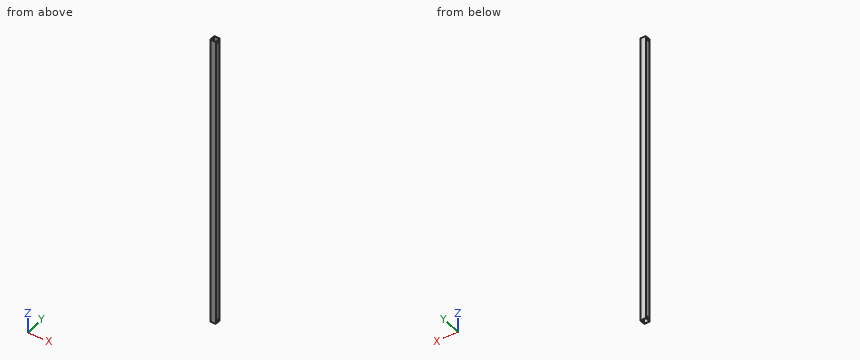
Autodesk Inventor part; units mm, degrees
ref_plane "YZ Plane" through (0, 0, 0) normal (1, 0, 0) x (0, 1, 0)
ref_plane "XZ Plane" through (0, 0, 0) normal (0, 1, 0) x (-1, 0, 0)
ref_plane "XY Plane" through (0, 0, 0) normal (0, 0, 1) x (1, 0, 0)
sketch "Sketch1" plane through (0, 0, 0) normal (0, 0, 1) x (1, 0, 0)
  line L0 (-12.7, 12.7) -> (12.7, 12.7)
  line L1 (12.7, 12.7) -> (12.7, -12.7)
  line L2 (12.7, -12.7) -> (-12.7, -12.7)
  line L3 (-12.7, -12.7) -> (-12.7, 12.7)
  line L4 (-17.78, 0) -> (17.78, 0)
  line L5 (0, 17.78) -> (0, -17.78)
  line L6 (11.43, 11.43) -> (-11.43, 11.43)
  line L7 (-11.43, 11.43) -> (-11.43, -11.43)
  line L8 (-11.43, -11.43) -> (11.43, -11.43)
  line L9 (11.43, -11.43) -> (11.43, 11.43)
  point P0 (0, 0)
  dimension "d0" = 25.4
  dimension "d1" = 1.27
extrude "Extrusion1" add sketch "Sketch1" along normal mid plane 1384.3 contours L0 L5 L6 L7 L4 L3 | L0 L1 L4 L9 L6 L5 | L4 L7 L8 L5 L2 L3 | L1 L2 L5 L8 L9 L4
sketch "Sketch2" plane through (12.7, 12.7, 692.15) normal (1, 0, 0) x (0, 0, -1)
  line L0 (0, 0) -> (1384.3, 0)
  line L1 (0, -25.4) -> (0, 0)
  line L2 (0, -25.4) -> (1384.3, -25.4)
  line L3 (1384.3, 0) -> (1384.3, -25.4)
  circle A0 centre (9.525, -12.7) radius 4.7625
  circle A1 centre (1374.775, -12.7) radius 4.7625
  line L4 (692.15, -30.48) -> (692.15, 5.08)
  point P0 (692.15, -12.7)
  dimension "d4" = 9.525
  dimension "d5" = 9.525
  dimension "d6" = 12.7
extrude "Extrusion2" cut sketch "Sketch2" against normal up to surface (25.4 mm away) contours A0 | A1
equation "\"d2\" = ArmLength"
equation "\"d7\" = ArmLength"
equation "\"ArmLength\" = 1384.3"
properties part number "Arm" material "Brass, Soft Yellow"
Model file for the job. Use its own axes, mm. Give positions to 0.01 mm unless a question says otherwise; leave off trailing zeros. Write each loop counter-clockwise with the first axis right and the second up, starting at its lowest first coordinate (ties: lowest second). Pieces come first, ordered by that corner, then holes. Notation, with made-up numbers: (-11, -24) -> (47, -24) arc R22 ccw to (47, -4) -> close; hole circle Ø2 at (-12.5, -36). An arc over 180 degrees is marked (long way). Write item = value, one per line.
(1) Slice it at B-B, the plane y = 0. Give the cut face in (x, z), then the cut area to 3 significant figures.
Determined:
outline = (-12.7, -692.15) -> (-11.43, -692.15) -> (-11.43, -687.39) -> (-12.7, -687.39) -> close; (-12.7, -677.86) -> (-11.43, -677.86) -> (-11.43, 677.86) -> (-12.7, 677.86) -> close; (-12.7, 687.39) -> (-11.43, 687.39) -> (-11.43, 692.15) -> (-12.7, 692.15) -> close; (11.43, -692.15) -> (12.7, -692.15) -> (12.7, -687.39) -> (11.43, -687.39) -> close; (11.43, -677.86) -> (12.7, -677.86) -> (12.7, 677.86) -> (11.43, 677.86) -> close; (11.43, 687.39) -> (12.7, 687.39) -> (12.7, 692.15) -> (11.43, 692.15) -> close
area = 3,470 mm2
(2) Slice it at A-A, the plane x = 2. Give the cut face in (y, z), then the cut area to 3 significant figures.
Determined:
outline = (-12.7, -692.15) -> (-11.43, -692.15) -> (-11.43, 692.15) -> (-12.7, 692.15) -> close; (11.43, -692.15) -> (12.7, -692.15) -> (12.7, 692.15) -> (11.43, 692.15) -> close
area = 3,520 mm2
(3) Slice it at C-C, the plane z = 438. Give the cut face in (x, y).
Determined:
outline = (-12.7, -12.7) -> (12.7, -12.7) -> (12.7, 12.7) -> (-12.7, 12.7) -> close; hole (-11.43, -11.43) -> (11.43, -11.43) -> (11.43, 11.43) -> (-11.43, 11.43) -> close
(4) Probe line 1 along X through (y, z) = (6.5, 233). List the from-to ranges inside material, lowest first.
Determined:
line_1 = -12.7 to -11.43, 11.43 to 12.7
